Could you check a few things on this drawing? It's one solid part, dimensions in mm from its lowest x, y, z. A direction names the side the tool comes from. Round coordinates to 2 decimals unless told otherwise and drop trailing zeros. Loops run counter-clockwise (first coordinate to the right, second up) from the corner with the lowest first, then second, coordinate; pieces in that order, holes last. Notation, with made-up numbers: M -3,48 L 53,48 A15 cw 53,63 Z; hole C 12.25,21.25 d2. An arc over 180 degrees is marked long. Use a Markdown table: item, result. Add a question column.
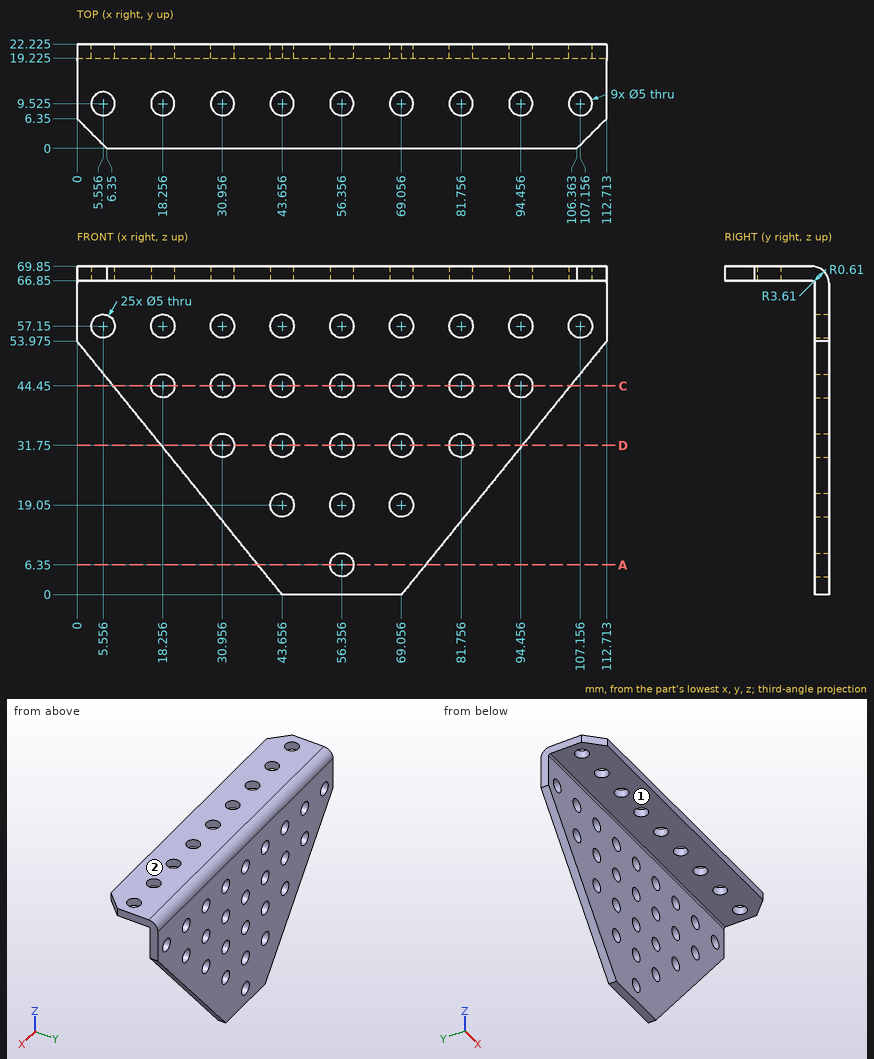
(1) Suppose I cut it at D-D on z = 31.75. List the corners of the cut face in (x, y) for me (1 decimal).
(2) Suppose I cut it at A-A on z = 6.35. List the corners of the cut face in (x, y) for me (1 decimal).
(3) On a 3-axis mill with a long thin cutter (end or side, diameter ignored), from which of +Z, -Z, +X, -X, +Y, -Y can I reach the whole of each face in a straight line? I mean the marked faces 1 and 2. Say none if no direction works.
(4) Suppose I cut it at C-C on z = 44.45. Count the separate pieces of the cut face and the enclosed holes in it, and give its area (3 significant figures).
(5) If I drill on probe 1 along Z at (x, y) = (94, 20) (1 decimal); probe 2 along Z at (x, y) = (97, 12); probe 3 along Y at (x, z) = (77, 18) (1 decimal), over which ranges is the centre line in solid material (lowest first)? Write a range as [from, to].
(6) I'm going to push flat-ended pins straight in: pin 1 (8 mm diameter, centred on x = 71, z = 51.5, fed in from -Y) (1 decimal); pin 2 (4.5 mm diameter, centred on x = 30.96, z = 57.15, fed in from -Y) (1 decimal); pin 3 (5 mm diameter, centred on x = 65.5, y = 7.5, fed in from -Z); pin 4 (10 mm diameter, centred on y = 16, z = 14.5, fed in from +X) (1 decimal). Where does each tip first touch, or does it pass through?
Results below:
| question | item | result |
|---|---|---|
| 1 | outline | M 18,19.2 L 28.5,19.2 L 28.5,22.2 L 18,22.2 Z; M 33.5,19.2 L 41.2,19.2 L 41.2,22.2 L 33.5,22.2 Z; M 46.2,19.2 L 53.9,19.2 L 53.9,22.2 L 46.2,22.2 Z; M 58.9,19.2 L 66.6,19.2 L 66.6,22.2 L 58.9,22.2 Z; M 71.6,19.2 L 79.3,19.2 L 79.3,22.2 L 71.6,22.2 Z; M 84.3,19.2 L 94.7,19.2 L 94.7,22.2 L 84.3,22.2 Z |
| 2 | outline | M 38.5,19.2 L 53.9,19.2 L 53.9,22.2 L 38.5,22.2 Z; M 58.9,19.2 L 74.2,19.2 L 74.2,22.2 L 58.9,22.2 Z |
| 3 | face 1 | -Z, +X, -X, -Y |
| 3 | face 2 | +Z, +X, -X, +Y, -Y |
| 4 | separate pieces | 8 |
| 4 | enclosed holes | 0 |
| 4 | area | 187 mm² |
| 5 | probe 1 | z = [30.8, 42], [46.9, 54.7], [59.6, 69.6] |
| 5 | probe 2 | z = [66.85, 69.85] |
| 5 | probe 3 | y = [19.2, 22.2] |
| 6 | pin 1 | stops at y = 19.2 |
| 6 | pin 2 | passes through |
| 6 | pin 3 | stops at z = 66.85 |
| 6 | pin 4 | stops at x = 83.9 |
